The model under review builds one solid part; all positions refer to its coordinate system, in mm. A direction names the side the tool comes from. Round coordinates to 2 decimals unless told otherwise and drop trailing zeros. Write each loop counter-clockwise with the first axis right and the second up, starting at its lowest first coordinate (ties: lowest second). Pieces come first, ordered by that corner, then holes. Notation, with made-up numbers: (-28, 68) - (8, 68) arc R11 cw to (8, 74) - close; hole circle Ø4 at (4.25, 12.5). An arc over 180 degrees is marked (long way). Return JSON: item names as keys, results as strings.
Solid Edge part; units mm, degrees
sketch "Sketch1" plane through (0, 0, 0) normal (0, 0, 1) x (1, 0, 0)
  line L0 (-25, -16) -> (25, -16)
  line L1 (25, -16) -> (25, 16)
  line L2 (25, 16) -> (-25, 16)
  line L3 (-25, 16) -> (-25, -16)
  dimension "D1" = 25
  dimension "D2" = 25
extrude "Protrusion1" add sketch "Sketch1" along normal blind 20
sketch "Sketch2" plane through (0, 0, 20) normal (0, 0, 1) x (0, 1, 0)
  line L0 (-10.25, 25) -> (10.25, 25)
  line L1 (10.25, 25) -> (10.25, -17.5)
  line L2 (10.25, -17.5) -> (-10.25, -17.5)
  line L3 (-10.25, -17.5) -> (-10.25, 25)
  dimension "D1" = 10.25
  dimension "D2" = 10.25
extrude "servo_cutout" cut sketch "Sketch2" against normal blind 14
hole "screw_bearing" at (7.5, 0, 0) direction (0, 0, 1) diameter 3.7 depth 30 tip angle 118 start chamfer 0.5 start chamfer angle 45 end chamfer 0.5 end chamfer angle 45
chamfer "Chamfer1" distance 0.5 angle 45 5 edges at (-3.75, -10.25, 20) (-25, -10.25, 13) (17.5, 0, 20) (-3.75, 10.25, 20) (-25, 10.25, 13)
hole "Hole1" at (-17.5, 13, 20) direction (0, 0, -1) diameter 2.8 depth 30 tip angle 118 start chamfer 0.3 start chamfer angle 45 end chamfer 0.3 end chamfer angle 45
hole "Hole2" at (-17.5, -13, 20) direction (0, 0, -1) diameter 2.8 depth 30 tip angle 118 start chamfer 0.3 start chamfer angle 45 end chamfer 0.3 end chamfer angle 45
chamfer "Chamfer2" distance 2 angle 45 3 edges at (-25, 0, 0) (-25, 16, 10) (-25, -16, 10)
fillet "Round1" radius 12 2 edges at (25, 16, 10) (25, -16, 10)
sketch "Sketch3" plane through (0, 0, 20) normal (0, 0, 1) x (0, 1, 0)
  line L0 (-6.25, 0) -> (6.25, 0)
  line L1 (6.25, 0) -> (6.25, -25)
  line L2 (6.25, -25) -> (-6.25, -25)
  line L3 (-6.25, -25) -> (-6.25, 0)
  dimension "D1" = 6.25
  dimension "D2" = 6.25
extrude "cable_cutout" cut sketch "Sketch3" against normal blind 12
chamfer "bottom_chamfer" distance 3 angle 45 5 edges at (21.4853, 12.4853, 0) (25, 0, 0) (21.4853, -12.4853, 0) (-5, -16, 0) (-5, 16, 0)
properties material "Polypropylene, general purpose"
(1) Add section D-D (x = -17.5). Write out the cut boundary in (y, z), plus the area to 3 significant figures.
Filled in:
{"outline": "(-16, 3) - (-14.4, 1.4) - (-14.4, 19.7) - (-14.7, 20) - (-16, 20) - close; (-11.6, 0.3) - (-11.3, 0) - (11.3, 0) - (11.6, 0.3) - (11.6, 19.7) - (11.3, 20) - (10.75, 20) - (10.25, 19.5) - (10.25, 6) - (-10.25, 6) - (-10.25, 19.5) - (-10.75, 20) - (-11.3, 20) - (-11.6, 19.7) - close; (14.4, 1.4) - (16, 3) - (16, 20) - (14.7, 20) - (14.4, 19.7) - close", "area": "233 mm2"}
(2) Add section C-C (y = 0). Write out the cut boundary in (x, z).
Filled in:
{"outline": "(-25, 2) - (-23, 0) - (5.15, 0) - (5.65, 0.5) - (5.65, 5.5) - (5.15, 6) - (-25, 6) - close; (9.35, 0.5) - (9.85, 0) - (22, 0) - (25, 3) - (25, 8) - (17.5, 8) - (17.5, 6) - (9.85, 6) - (9.35, 5.5) - close"}
(3) Add section B-B (x = 7.5). Write out the cut boundary in (y, z), plus the area to 3 significant figures.
Filled in:
{"outline": "(-16, 3) - (-13, 0) - (-2.35, 0) - (-1.85, 0.5) - (-1.85, 5.5) - (-2.35, 6) - (-10.25, 6) - (-10.25, 19.5) - (-10.75, 20) - (-16, 20) - close; (1.85, 0.5) - (2.35, 0) - (13, 0) - (16, 3) - (16, 20) - (10.75, 20) - (10.25, 19.5) - (10.25, 6) - (2.35, 6) - (1.85, 5.5) - close", "area": "321 mm2"}
(4) Wall thickness on line 1 (Y direction, x = -17.5, z = 12); line 2 (Y direction, x = -20, z = 12.5); line 3 (Y direction, x = -17, z = 10.75): over which ranges is each line inside the solid? List them lowest first.
Filled in:
{"line 1": "y = -16 to -14.4, -11.6 to -10.25, 10.25 to 11.6, 14.4 to 16", "line 2": "y = -16 to -10.25, 10.25 to 16", "line 3": "y = -16 to -14.31, -11.69 to -10.25, 10.25 to 11.69, 14.31 to 16"}
(5) For faces 4 (the flat face through (-4, 10.25, 13)), 5 (the conical face through (19.89, -11.04, 0.85)), list the 3-axis set-ups (+Z, -Z, +X, -X, +Y, -Y) from which the entire face can be reached by the end or side of a thin tool; tool diameter is ignored.
Filled in:
{"face 4": "+Z, -X", "face 5": "-Z, +X, -Y"}
(6) Clearance check with flat-ended pins moving along their axes: pin 1 Ø4.5 at (x, y) = (7.5, 0) entering from -Z; pin 2 Ø4 at (x, y) = (-18.5, 4.5) entering from +Z; pin 3 Ø10 at (x, z) = (20, 4) entering from +Y. State where each tip first meets the part, or that it passes through.
Filled in:
{"pin 1": "stops at z = 0.1", "pin 2": "stops at z = 6", "pin 3": "stops at y = 15.83"}
(7) Mouldability with a two-part tool opening along X and no side actions: class faces 1 (the conical face through (-17.46, 11.48, 0.18)), 2 (the flat face through (21, 0, 8)), 3 (the cylindrical face through (21.58, 12.39, 11.62)) as released by +X, released by -X, zero draft, split by the parting line, or undercut.
Filled in:
{"face 1": "undercut", "face 2": "zero draft", "face 3": "released by +X"}
(8) Add section A-A (z = 14.75). Write out the cut boundary in (x, y).
Filled in:
{"outline": "(-25, -14) - (-23, -16) - (13, -16) arc R12 ccw to (24.79, -6.25) - (17.5, -6.25) - (17.5, -10.25) - (-24.5, -10.25) - (-25, -10.75) - close; (-25, 10.75) - (-24.5, 10.25) - (17.5, 10.25) - (17.5, 6.25) - (24.79, 6.25) arc R12 ccw to (13, 16) - (-23, 16) - (-25, 14) - close; hole circle Ø2.8 at (-17.5, -13); hole circle Ø2.8 at (-17.5, 13)"}
